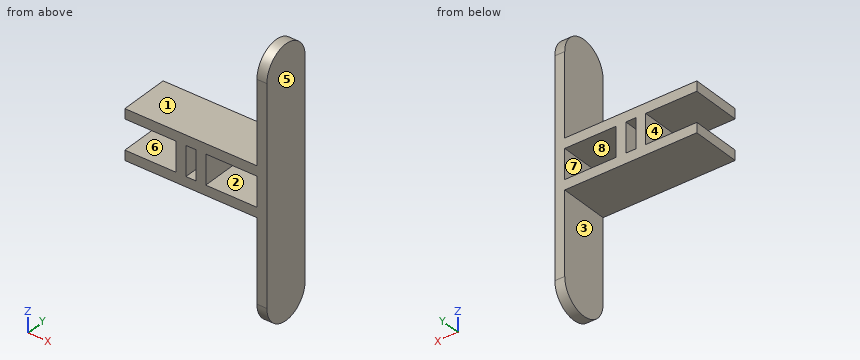
Autodesk Inventor part; units mm, degrees
ref_plane "Work Plane1" through (0, 0, 6) normal (0, 0, 1) x (1, 0, 0)
ref_plane "Work Plane2" through (0, 15, -6) normal (0, 0, -1) x (-1, 0, 0)
ref_plane "XZ Plane" through (0, 0, 0) normal (0, 1, 0) x (-1, 0, 0)
sketch "Sketch1" plane through (0, 0, 0) normal (1, 0, 0) x (0, 1, 0)
  line L0 (15, 0) -> (15, 32.5)
  line L1 (15, 6) -> (0, 6)
  line L2 (0, 32.5) -> (0, 0)
  line L3 (15, 0) -> (15, 32.5)
  line L4 (15, 6) -> (0, 6)
  line L5 (0, 32.5) -> (0, 0)
  arc A0 (15, 32.5) -> (0, 32.5) centre (7.5, 32.5) ccw
  line L6 (15, 0) -> (0, 0)
  line L7 (15, 0) -> (15, -32.5)
  line L8 (15, -6) -> (0, -6)
  line L9 (0, -32.5) -> (0, 0)
  line L10 (15, -6) -> (0, -6)
  line L11 (15, 0) -> (15, -32.5)
  line L12 (0, -32.5) -> (0, 0)
  arc A1 (0, -32.5) -> (15, -32.5) centre (7.5, -32.5) ccw
  dimension "d25" = 65
  dimension "d26" = 15
ref_plane "Work Plane1" through (0, 0, 6) normal (0, 0, 1) x (1, 0, 0)
ref_plane "Work Plane2" through (0, 15, -6) normal (0, 0, -1) x (-1, 0, 0)
extrude "Extrusion1" add sketch "Sketch1" along normal mid plane 3
sketch "Sketch2" plane through (0, 0, 6) normal (0, 0, 1) x (1, 0, 0)
  line L0 (-1.5, 15) -> (-41.5, 15)
  line L1 (-41.5, 15) -> (-41.5, 0)
  line L2 (-41.5, 0) -> (-1.5, 0)
  line L3 (-21.5, 15) -> (-21.5, 0)
  line L4 (-18.5, 15) -> (-18.5, 0)
  line L5 (-24.5, 15) -> (-24.5, 0)
  line L6 (-1.5, 15) -> (-1.5, 0)
  line L7 (-1.5, 0) -> (0, 0)
  dimension "d30" = 40
  dimension "d31" = 3
  dimension "d32" = 3
sketch "Sketch3" plane through (0, 15, -6) normal (0, 0, -1) x (-1, 0, 0)
  line L0 (1.5, -15) -> (1.5, 0)
  line L1 (41.5, 0) -> (41.5, -15)
  line L2 (41.5, -15) -> (1.5, -15)
  line L3 (1.5, 0) -> (41.5, 0)
  line L4 (21.5, 0) -> (21.5, -15)
  line L5 (24.5, 0) -> (24.5, -15)
  line L6 (18.5, 0) -> (18.5, -15)
  line L7 (1.5, 0) -> (1.5, -15)
  point P0 (0, -15)
  dimension "d35" = 40
ref_plane "Work Plane5" through (-18.5, 0, 0) normal (1, 0, 0) x (0, 1, 0)
ref_plane "Work Plane6" through (-24.5, 15, 6) normal (1, 0, 0) x (0, 1, 0)
ref_plane "Work Plane7" through (-41.5, 15, 6) normal (1, 0, 0) x (0, 1, 0)
sketch "Sketch5" plane through (-18.5, 0, 0) normal (1, 0, 0) x (0, 1, 0)
  line L0 (15, -32.5) -> (15, 32.5)
  line L1 (0, 0) -> (15, 0)
  line L2 (15, 0) -> (15, 6)
  line L3 (15, 6) -> (0, 6)
  line L4 (0, 6) -> (0, 0)
  line L5 (0, 0) -> (15, 0)
  line L6 (15, 0) -> (15, -6)
  line L7 (15, -6) -> (0, -6)
  line L8 (0, -6) -> (0, 0)
  dimension "d42" = 6
  dimension "d43" = 6
sketch "Sketch6" plane through (-24.5, 15, 6) normal (1, 0, 0) x (0, 1, 0)
  line L0 (-15, -6) -> (0, -6)
  line L1 (0, -6) -> (0, 0)
  line L2 (0, 0) -> (-15, 0)
  line L3 (-15, 0) -> (-15, -6)
  line L4 (0, -38.5) -> (0, 26.5)
  line L5 (-15, -6) -> (0, -6)
  line L6 (0, -6) -> (0, -12)
  line L7 (0, -12) -> (-15, -12)
  line L8 (-15, -12) -> (-15, -6)
  dimension "d44" = 6
extrude "Extrusion2" add sketch "Sketch2" along normal mid plane 3
extrude "Extrusion3" add sketch "Sketch3" along normal mid plane 3
extrude "Extrusion4" add sketch "Sketch6" along normal mid plane 3
extrude "Extrusion5" add sketch "Sketch5" along normal mid plane 3
properties part number "LegMiddle"
Input: part model. Units: mm. Frame: model coordinates. Face numbers are marked on the shaded views. A direction names the side the tool comes from. Coordinates: 2 decimals unless noted, no trailing zeros. Loops run counter-clockwise (first coordinate to the right, second up) from the corner with the lowest first, then second, coordinate; pieces in that order, holes last.
(1) Section B-B on x = -28.5. Return the cut outline in (y, z).
(2) Section A-A on y = 13.5. Return the cut outline in (x, z).
(3) Material intervals for probe 1 along X at (y, z) = (14.25, 0); probe 2 along Z at (x, y) = (-8.5, 8.75); probe 3 along X at (y, z) = (8, -28), sorted ascending.
(4) First-contact query: pin 1 Ø4.5 at (x, y) = (-30.5, 10) entering from +Z; pin 2 Ø7.5 at (x, y) = (-24, 6.5) entering from -Z; pin 3 Ø2.5 at (y, z) = (4.5, -1.5) entering from -X. Flat tips, straight axial feed; report the tip coordinate or a pass-through.
(5) Pull-direction query (X, two-part tool) for the marked faces 5, 6, 7 and 8; classes: released by +X, released by -X, zero draft, split by the parting line, or undercut.
(6) Set-up query: the marked faces 1, 2, 3 and 4. Return all of +Z, -Z, +X, -X, +Y, -Y with unobstructed straight access to the full face (end or side cutting, diameter ignored); none if empty.
(7) Section C-C on z = -15. Return the cut outline in (x, y), then the cut area to 3 significant figures.
(8) Section D-D on y = 7.5. Return the cut outline in (x, z).
Data:
1. outline: (0, -7.5) - (15, -7.5) - (15, -4.5) - (0, -4.5) - close; (0, 4.5) - (15, 4.5) - (15, 7.5) - (0, 7.5) - close
2. outline: (-41.5, -7.5) - (-1.5, -7.5) - (-1.5, -37) - (1.5, -37) - (1.5, 37) - (-1.5, 37) - (-1.5, 7.5) - (-41.5, 7.5) - (-41.5, 4.5) - (-26, 4.5) - (-26, -4.5) - (-41.5, -4.5) - close; hole (-23, -4.5) - (-20, -4.5) - (-20, 4.5) - (-23, 4.5) - close; hole (-17, -4.5) - (-1.5, -4.5) - (-1.5, 4.5) - (-17, 4.5) - close
3. probe 1: x = -26 to -23, -20 to -17, -1.5 to 1.5
3. probe 2: z = -7.5 to -4.5, 4.5 to 7.5
3. probe 3: x = -1.5 to 1.5
4. pin 1: stops at z = 7.5
4. pin 2: stops at z = -7.5
4. pin 3: stops at x = -26
5. face 5: released by +X
5. face 6: zero draft
5. face 7: undercut
5. face 8: undercut
6. face 1: +Z, -X, +Y, -Y
6. face 2: +Y, -Y
6. face 3: -Z, -X, +Y, -Y
6. face 4: -X, +Y, -Y
7. outline: (-1.5, 0) - (1.5, 0) - (1.5, 15) - (-1.5, 15) - close
7. area: 45.0 mm2
8. outline: (-41.5, -7.5) - (-1.5, -7.5) - (-1.5, -40) - (1.5, -40) - (1.5, 40) - (-1.5, 40) - (-1.5, 7.5) - (-41.5, 7.5) - (-41.5, 4.5) - (-26, 4.5) - (-26, -4.5) - (-41.5, -4.5) - close; hole (-23, -4.5) - (-20, -4.5) - (-20, 4.5) - (-23, 4.5) - close; hole (-17, -4.5) - (-1.5, -4.5) - (-1.5, 4.5) - (-17, 4.5) - close
